Can you work these out from the model? Positions are in its coordinate system, mm. Face numbers are marked on the shaded views. A direction names the side the tool comes from. Coordinates: 2 decimals unless noted, no trailing zeros. Order: outer loops, then holes, each group sorted by start corner. A loop starts at its lowest first (then second) coordinate and runs counter-clockwise, first axis right, second up. Notation, with made-up numbers: (74, -33.5) -> (103, -33.5) arc R20 cw to (103, 2.5) -> close; hole circle Ø10 at (82, 5). An arc over 180 degrees is marked (long way). Answer as CSV lines item,"result".
from build123d import *

# Parameters (mm, degrees)
F1_DEPTH    = 10
F2_R        = 2.65
F2_R_2      = 2.7
F3_DEPTH    = 10.001
F4_T2_ANGLE = 6.3743045961
F6_DEPTH    = 6
F7_R        = 2
F8_T1_DEPTH = 17.7150489639
F8_T3_DEPTH = 16.827176909
F8_T5_DEPTH = 14.1871505468
F9_T1_DEPTH = 16.8101610382
F10_R       = 2
F11_DEPTH   = 16


# Not quite as in the source:
# - a fillet or chamfer that OpenCascade refuses, or shapes differently, is made with other operations: its cross-section is extruded or revolved along the edge and cut away or added
# - a feature names something its author has since deleted; it is built from what else it names


with BuildPart() as f1:
    # F0 (on Top) → F1 (new body)
    with BuildSketch(Plane.XY):
        with BuildLine():
            Line((-34.7499609253, -11.2477834763), (-54.7499609253, -11.1477834763))
            Line((-54.7499609253, -11.1477834763), (-54.8004609253, -21.2477834763))
            Line((-54.8004609253, -21.2477834763), (-42.8006109225, -21.3077827264))
            ThreePointArc((-42.8006109225, -21.3077827264), (-20.5885311059, -33.3218659489), (-10, -56.2477834763))
            Line((-10, -56.2477834763), (0, -56.2477834763))
            ThreePointArc((0, -56.2477834763), (0.1673692192, -47.7484327866), (0.2444140549, -39.2477834763))
            Line((0.2444140549, -39.2477834763), (-0.07466726, -32.2477834763))
            ThreePointArc((-0.07466726, -32.2477834763), (-4.6744272783, -21.4152799032), (-13.7499609253, -13.9229094565))
            Line((-13.7499609253, -13.9229094565), (-22.7499609253, -12.1477834763))
            ThreePointArc((-22.7499609253, -12.1477834763), (-28.7364107349, -11.5171142711), (-34.7499609253, -11.2477834763))
        make_face()
    extrude(amount=F1_DEPTH)

    # F2 (on face) → F3 (cut, through all)
    with BuildSketch(Plane.XY.offset(10)):
        with Locations((-47.7499609253, -17.1477834763)):
            Circle(F2_R)
        with Locations((-17.7499609253, -21.2477834763)):
            Circle(F2_R)
        with Locations((-7.7499609253, -50.2477834763)):
            Circle(F2_R)
        with Locations((-7.7499609253, -30.2477834763)):
            Circle(F2_R_2)
    extrude(amount=-F3_DEPTH, mode=Mode.SUBTRACT)

    # F4: fillet of radius 6 on 1 edges, made by hand

    # F4_s1 → F4_t2 (revolve, cut)
    with BuildSketch(Plane(origin=(-6.441827323, -91.8723118046, 0), x_dir=(0, 0, 1), z_dir=(-0.0699454492, -0.9975508178, 0))):
        with BuildLine():
            ThreePointArc((0, 1.2558600799), (1.7573593129, -2.9867806073), (6, -4.7441399201))
            Line((6, -4.7441399201), (6, -4.8641399201))
            Line((6, -4.8641399201), (-0.12, -4.8641399201))
            Line((-0.12, -4.8641399201), (-0.12, 1.2558600799))
            Line((-0.12, 1.2558600799), (0, 1.2558600799))
        make_face()
    revolve(axis=Axis((-799.7499609255, -36.2477834763, 0), (0, 0, 1)), revolution_arc=F4_T2_ANGLE, mode=Mode.SUBTRACT)

    # F5 (on face) → F6 (join)
    with BuildSketch(Plane.XY):
        Polygon((-20, -32.2477834763), (-14.04, -41.3386925673), (-9.04, -42.2477834763), (-9, -34.2477834763), align=None)
    extrude(amount=-F6_DEPTH)

    # F7
    f7_edges = [f1.edges().sort_by_distance(p)[0] for p in [
        (-9, -34.247783, -3),
        (-20, -32.247783, -3),
        (-14.04, -41.338693, -3),
        (-9.04, -42.247783, -3),
    ]]
    fillet(f7_edges, radius=F7_R)

    # F8: chamfer of 1.5 on 4 edges, made by hand

    # F8_s2 → F8_t1 (cut)
    with BuildSketch(Plane.XY.offset(-3.8575244819)):
        Polygon((-53.2499796749, -11.1552833826), (-54.7574608315, -12.6477647267), (-54.7499609253, -11.1477834763), align=None)
        Polygon((-54.792961019, -19.747802226), (-53.3004796749, -21.2552833826), (-54.8004609253, -21.2477834763), align=None)
    extrude(amount=F8_T1_DEPTH, mode=Mode.SUBTRACT)

    # F8_s4 → F8_t3 (cut)
    with BuildSketch(Plane.XY.offset(-3.4135884545)):
        with BuildLine():
            Line((-10.1649915082, -54.9628953089), (-8.6804960049, -56.2477834763))
            Line((-8.6804960049, -56.2477834763), (-10, -56.2477834763))
            ThreePointArc((-10, -56.2477834763), (-10.0801500361, -55.5824778984), (-10.1649915082, -54.9628953089))
        make_face()
    extrude(amount=F8_T3_DEPTH, mode=Mode.SUBTRACT)

    # F8_s6 → F8_t5 (cut)
    with BuildSketch(Plane.XY.offset(-0.4141318258)):
        with BuildLine():
            Line((-1.4642977695, -56.2477834763), (0.0352995939, -54.7825361376))
            ThreePointArc((0.0352995939, -54.7825361376), (0.0185023043, -55.4936979353), (0, -56.2477834763))
            Line((0, -56.2477834763), (-1.4642977695, -56.2477834763))
        make_face()
    extrude(amount=F8_T5_DEPTH, mode=Mode.SUBTRACT)

    # F9: chamfer of 1 on 1 edges, made by hand

    # F9_s2 → F9_t1 (cut)
    with BuildSketch(Plane.XY.offset(-3.4050805191)):
        with BuildLine():
            Line((-12.5377780347, -14.5439926831), (-14.8624749797, -13.6972040173))
            Line((-14.8624749797, -13.6972040173), (-14.8586048158, -13.6775820441))
            ThreePointArc((-14.8586048158, -13.6775820441), (-14.3029436702, -13.7934559205), (-13.7460907615, -13.9032874834))
            Line((-13.7460907615, -13.9032874834), (-13.7412512479, -13.9049055259))
            ThreePointArc((-13.7412512479, -13.9049055259), (-13.1317908034, -14.2101386142), (-12.5281211003, -14.5264785854))
            Line((-12.5281211003, -14.5264785854), (-12.5377780347, -14.5439926831))
        make_face()
    extrude(amount=F9_T1_DEPTH, mode=Mode.SUBTRACT)

    # F10 (on face) → F11 (cut, through all)
    with BuildSketch(Plane(origin=(0, 0, -6), x_dir=(1, 0, 0), z_dir=(0, 0, -1))):
        with Locations((-12.50838816, 37.9476757883)):
            Circle(F10_R)
    extrude(amount=-F11_DEPTH, mode=Mode.SUBTRACT)


solid = f1.part
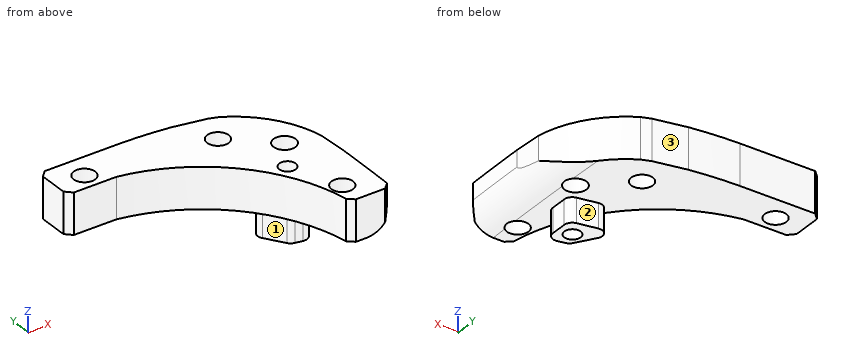
Q1. If I drill on line 1 (Y direction, x = -8, z = 4.75); line 2 (Y direction, x = -46, z = 6); line 3 (X direction, y = -53.5, z = 5.5), over which ranges is the centre line in solid material (lowest first)?
Solution:
line 1,"-56.25 to -52.89, -47.61 to -32.94, -27.56 to -17.78"
line 2,"-21.29 to -19.14, -15.16 to -11.19"
line 3,"-10.4 to 0.04"
Q2. Imagine slicing it at C-C (x = -28). List the corners of the cut face in (y, z) for me.
Solution:
outline,"(-27.13, 0) -> (-11.58, 0) -> (-11.58, 10) -> (-27.13, 10) -> close"
Q3. Imagine slicing it at A-A (z = -3.25). List the corners of the cut face in (x, y) for me, and give its area (3 significant figures).
Solution:
outline,"(-17.44, -36.15) -> (-14.51, -40.62) arc R2 ccw to (-13.2, -41.49) -> (-11.39, -41.82) arc R2 ccw to (-9.03, -39.86) -> (-9.01, -35.93) arc R2 ccw to (-10.65, -33.95) -> (-15.41, -33.08) arc R2 ccw to start; hole circle Ø4 at (-12.51, -37.95)"
area,"44.9 mm2"
Q4. For P1, Ø6, axis at x = -7.75, y = -50.25, coming from the -Z side; P2, Ø5, axis at y = -34.5, z = 0.5, coming from the +X side; P3, Ø8, axis at x = -23.5, z = -3, coming from the -Y side; P4, Ø4, axis at x = -47.75, y = -17.15, coming from the +Z side, each with a flat end and sliding along its axis, tell me the tip position at first contact or that it passes through.
Solution:
P1,"z = 0"
P2,"x = -0.56"
P3,"y = -33.04"
P4,"through"
Q5. Which directions (+Z, -Z, +X, -X, +Y, -Y) give clear straight access to the entire face, cutting with the end or side of a thin tool? Please do the marked faces 1, 2 and 3.
Solution:
face 1,"-Z, -X, -Y"
face 2,"-Z, +X, +Y"
face 3,"+Z, -Z, +X, +Y"
Q6. Imagine slicing it at B-B (z = 3). Give the number of separate pieces and of enclosed holes in the cut face, and give its area (3 significant figures).
Solution:
separate pieces,"1"
enclosed holes,"5"
area,"953 mm2"
